The listing builds one solid part. Answer for the finished solid, in the listing's coordinates (mm). A direction names the side the tool comes from. Coordinates: 2 decimals unless noted, no trailing zeros. Order: outer loops, then holes, each group sorted by start corner. A loop starts at its lowest first (then second) coordinate and runs counter-clockwise, first axis right, second up. Notation, with made-up numbers: M 89.5,81.5 L 102.5,81.5 A12 ccw 102.5,89.5 Z; hole C -35.75,44 d2. An arc over 180 degrees is marked long. One line per item, written item: value. Start each with the question number.
Q1. The part is cut by section D-D on y = -0.8. Give the number of separate pieces and of enclosed holes in the cut face, then the cut area to 3 significant figures.
Q2. The part is cut by section A-A on x = -17.8. Give the vertices of the cut face in (y, z).
Q3. For faces 1 (the flat face through (13.55, -1, 19)), 2 (the flat face through (13.55, -1, -19)), 3 (the flat face through (-12.28, -0.69, 14.16)), 4 (the flat face through (-4.25, -1, -19)), 5 (the cylindrical face through (-19.95, -0.71, -17.33)), determine the directions among +Z, -Z, +X, -X, +Y, -Y from which every point of the face is accessible in a straight line to the end or side of a thin tool.
Q4. This flat-tipped pin is pushed along its axis until it touches: pin 1 Ø0.7 at (y, z) = (-0.5, 19.5) entering from +X. Where does it stop, or does it pass through?
Q5. The part is cut by section C-C on x = -12.5. Give the vertices of the cut face in (y, z).
Q6. The part is cut by section B-B on z = 1.5. Give the vertices of the cut face in (x, y) (3 decimals), then the cut area to 3 significant figures.
Q7. Straight lines are drawn through the part: line 1 along X through (y, z) = (-1, 0) (3 decimals); line 2 along X through (y, z) = (-1.1, 11); line 3 along X through (y, z) = (-0.4, 15.15). For each, find the intervals that lie inside material, in ascending order. Write a range as [from, to].
Q8. Determine the mould class of faces 6 (the cylindrical face through (-14.63, -0.71, -7.4)), 7 (the flat face through (12.26, -0.69, 14.14)), 8 (the flat face through (-0.3, -1.4, 14.2)), 9 (the flat face through (17, -1, 17.9)) for opening direction Z: pulls with the +Z half, pulls with the -Z half, needs draft (parallel to the pull), parting line crosses it, or undercut.
```python
from build123d import *

# Parameters (mm, degrees)
F0_R     = 1.5
F0_W     = 9.3
F0_H     = 2.9
F1_DEPTH = 1.4
F2_R     = 4
F3_DEPTH = 2
F4_R     = 2


# Not quite as in the source:
# - a pattern or mirror of a feature is missing from the dataset's text; its kind, count and spacing are read off the source's solid
# - a feature names something its author has since deleted; it is built from what else it names


with BuildPart() as f1:
    # F0 (on Front) → F1 (new body)
    with BuildSketch(Plane.XZ):
        with BuildLine():
            Line((15.55, -17.9), (20.55, -17.9))
            Line((20.55, -17.9), (20.55, 17.9))
            Line((20.55, 17.9), (15.55, 17.9))
            ThreePointArc((15.55, 17.9), (14.55, 16.9), (13.55, 17.9))
            Line((13.55, 17.9), (4.25, 17.9))
            ThreePointArc((4.25, 17.9), (3.25, 16.9), (2.25, 17.9))
            Line((2.25, 17.9), (-2.25, 17.9))
            ThreePointArc((-2.25, 17.9), (-3.25, 16.9), (-4.25, 17.9))
            Line((-4.25, 17.9), (-13.55, 17.9))
            ThreePointArc((-13.55, 17.9), (-14.55, 16.9), (-15.55, 17.9))
            Line((-15.55, 17.9), (-20.55, 17.9))
            Line((-20.55, 17.9), (-20.55, -17.9))
            Line((-20.55, -17.9), (-15.55, -17.9))
            ThreePointArc((-15.55, -17.9), (-14.55, -16.9), (-13.55, -17.9))
            Line((-13.55, -17.9), (-4.25, -17.9))
            ThreePointArc((-4.25, -17.9), (-3.25, -16.9), (-2.25, -17.9))
            Line((-2.25, -17.9), (2.25, -17.9))
            ThreePointArc((2.25, -17.9), (3.25, -16.9), (4.25, -17.9))
            Line((4.25, -17.9), (13.55, -17.9))
            ThreePointArc((13.55, -17.9), (14.55, -16.9), (15.55, -17.9))
        make_face()
        with BuildLine():
            ThreePointArc((-13.1202274148, -14.9978997242), (-15.343659863, -14.8848474001), (-15.0056689733, -12.6843486297))
            Line((-15.0056689733, -12.6843486297), (-13.3106601718, -10.9893398282))
            ThreePointArc((-13.3106601718, -10.9893398282), (-11.6759748515, -10.6641807012), (-10.75, -12.05))
            ThreePointArc((-10.75, -12.05), (-10.8131046691, -12.4805018095), (-10.9971090773, -12.8747813867))
            ThreePointArc((-10.9971090773, -12.8747813867), (-11.1893398282, -13.1106601718), (-11.4252186133, -13.3028909227))
            Line((-11.4252186133, -13.3028909227), (-13.1202274148, -14.9978997242))
        make_face(mode=Mode.SUBTRACT)
        with BuildLine():
            Line((13.3106601718, -10.9893398282), (15.0056689733, -12.6843486297))
            ThreePointArc((15.0056689733, -12.6843486297), (15.5013367677, -13.2256118689), (15.6808875866, -13.9372395524))
            ThreePointArc((15.6808875866, -13.9372395524), (14.7549127351, -15.3230588512), (13.1202274148, -14.9978997242))
            Line((13.1202274148, -14.9978997242), (11.4252186133, -13.3028909227))
            ThreePointArc((11.4252186133, -13.3028909227), (11.1893398282, -13.1106601718), (10.9971090773, -12.8747813867))
            ThreePointArc((10.9971090773, -12.8747813867), (11.3023921523, -10.8872277235), (13.3106601718, -10.9893398282))
        make_face(mode=Mode.SUBTRACT)
        with Locations((-17.8, 15.15)):
            Circle(F0_R, mode=Mode.SUBTRACT)
        with BuildLine():
            ThreePointArc((-15.0056689733, 12.6843486297), (-15.343659863, 14.8848474001), (-13.1202274148, 14.9978997242))
            Line((-13.1202274148, 14.9978997242), (-11.4252186133, 13.3028909227))
            ThreePointArc((-11.4252186133, 13.3028909227), (-11.1893398282, 13.1106601718), (-10.9971090773, 12.8747813867))
            ThreePointArc((-10.9971090773, 12.8747813867), (-10.8131046691, 12.4805018095), (-10.75, 12.05))
            ThreePointArc((-10.75, 12.05), (-11.6759748515, 10.6641807012), (-13.3106601718, 10.9893398282))
            Line((-13.3106601718, 10.9893398282), (-15.0056689733, 12.6843486297))
        make_face(mode=Mode.SUBTRACT)
        with BuildLine():
            ThreePointArc((-10.9201648339, 8.6), (0, 13.9), (10.9201648339, 8.6))
            Line((10.9201648339, 8.6), (15.775, 8.6))
            Line((15.775, 8.6), (15.775, -8.6))
            Line((15.775, -8.6), (10.9201648339, -8.6))
            ThreePointArc((10.9201648339, -8.6), (0, -13.9), (-10.9201648339, -8.6))
            Line((-10.9201648339, -8.6), (-15.775, -8.6))
            Line((-15.775, -8.6), (-15.775, 8.6))
            Line((-15.775, 8.6), (-10.9201648339, 8.6))
        make_face(mode=Mode.SUBTRACT)
        with BuildLine():
            ThreePointArc((13.1202274148, 14.9978997242), (14.7549127351, 15.3230588512), (15.6808875866, 13.9372395524))
            ThreePointArc((15.6808875866, 13.9372395524), (15.5013367677, 13.2256118689), (15.0056689733, 12.6843486297))
            Line((15.0056689733, 12.6843486297), (13.3106601718, 10.9893398282))
            ThreePointArc((13.3106601718, 10.9893398282), (11.3023921523, 10.8872277235), (10.9971090773, 12.8747813867))
            ThreePointArc((10.9971090773, 12.8747813867), (11.1893398282, 13.1106601718), (11.4252186133, 13.3028909227))
            Line((11.4252186133, 13.3028909227), (13.1202274148, 14.9978997242))
        make_face(mode=Mode.SUBTRACT)
        with Locations((-8.9, -19.35)):
            Rectangle(F0_W, F0_H)
        with Locations((8.9, -19.35)):
            Rectangle(F0_W, F0_H)
        with Locations((8.9, 19.35)):
            Rectangle(F0_W, F0_H)
    extrude(amount=F1_DEPTH)

    # F1_copies: F1 across plane


with BuildPart() as f1_1:
    add(f1.part)
    add(f1.part.mirror(Plane.XY))

    # F2
    f2_edges = [f1_1.edges().sort_by_distance(p)[0] for p in [
        (-15.775, -0.7, 8.6),
        (-15.775, -0.7, -8.6),
        (15.775, -0.7, 8.6),
        (15.775, -0.7, -8.6),
    ]]
    fillet(f2_edges, radius=F2_R)

    # F0 (on Front) → F3 (cut)
    with BuildSketch(Plane.XZ):
        with BuildLine():
            ThreePointArc((-4.25, 17.9), (-3.25, 16.9), (-2.25, 17.9))
            Line((-2.25, 17.9), (-4.25, 17.9))
        make_face()
        with BuildLine():
            Line((-4.25, 17.9), (-2.25, 17.9))
            ThreePointArc((-2.25, 17.9), (-3.25, 18.9), (-4.25, 17.9))
        make_face()
        with Locations((-17.8, 15.15)):
            Circle(F0_R)
    extrude(amount=F3_DEPTH, mode=Mode.SUBTRACT)

    # F4
    f4_edges = [f1_1.edges().sort_by_distance(p)[0] for p in [
        (-20.55, -0.7, 17.9),
        (20.55, -0.7, 17.9),
        (20.55, -0.7, -17.9),
        (-20.55, -0.7, -17.9),
    ]]
    fillet(f4_edges, radius=F4_R)


solid = f1_1.part
```
Output:
1. separate pieces: 1
1. enclosed holes: 6
1. area: 805 mm^2
2. outline: M -1.4,-17.9 L 0,-17.9 L 0,13.65 L -1.4,13.65 Z; M -1.4,16.65 L 0,16.65 L 0,17.9 L -1.4,17.9 Z
3. face 1: +Z, +X, +Y, -Y
3. face 2: -Z, +X, +Y, -Y
3. face 3: +Y, -Y
3. face 4: -Z, +Y, -Y
3. face 5: -Z, -X, +Y, -Y
4. pin 1: stops at x = 13.55
5. outline: M -1.4,-20.8 L 0,-20.8 L 0,-14.38 L -1.4,-14.38 Z; M -1.4,-10.57 L 0,-10.57 L 0,-8.53 L -1.4,-8.53 Z; M -1.4,8.53 L 0,8.53 L 0,10.57 L -1.4,10.57 Z; M -1.4,14.38 L 0,14.38 L 0,20.8 L -1.4,20.8 Z
6. outline: M -20.55,-1.4 L -15.775,-1.4 L -15.775,0 L -20.55,0 Z; M 15.775,-1.4 L 20.55,-1.4 L 20.55,0 L 15.775,0 Z
6. area: 13.4 mm^2
7. line 1: x = [-20.55, -15.775], [15.775, 20.55]
7. line 2: x = [-20.55, -13.32], [-11.18, -8.5], [8.5, 11.18], [13.32, 20.55]
7. line 3: x = [-20.55, -19.3], [-16.3, -15.06], [-13.3, 13.3], [15.06, 20.55]
8. face 6: undercut
8. face 7: undercut
8. face 8: needs draft
8. face 9: pulls with the +Z half
